Geometry: final body of the model. Coordinates: model frame, mm. Face numbers are marked on the shaded views. A direction names the side the tool comes from. Coordinates: 2 decimals unless noted, no trailing zeros. Order: outer loops, then holes, each group sorted by start corner. A loop starts at its lowest first (then second) coordinate and runs counter-clockwise, first axis right, second up. Notation, with made-up numbers: (51, 73.5) - (66, 73.5) arc R16 cw to (66, 86.5) - close; hole circle Ø11 at (-33.75, 26). An arc over 180 degrees is marked (long way). Use a Markdown table: item, result. Add a question column.
```python
from build123d import *

# Parameters (mm, degrees)
SKETCH1_W           = 50
SKETCH1_H           = 25
BOSS_EXTRUDE1_DEPTH = 25
SKETCH2_W           = 37
SKETCH2_H           = 21
CUT_EXTRUDE1_DEPTH  = 11
SKETCH3_W           = 3
SKETCH3_H           = 21
CUT_EXTRUDE2_DEPTH  = 8
SKETCH7_W           = 25
SKETCH7_H           = 25
BOSS_EXTRUDE2_DEPTH = 19
CUT_EXTRUDE3_DEPTH  = 13
SKETCH10_W          = 25
SKETCH10_H          = 25
BOSS_EXTRUDE3_DEPTH = 10
CUT_EXTRUDE5_DEPTH  = 25


with BuildPart() as part:
    # Sketch1 → Boss-Extrude1 (new body)
    with BuildSketch(Plane.XY):
        with Locations((-5, 0)):
            Rectangle(SKETCH1_W, SKETCH1_H)
    extrude(amount=BOSS_EXTRUDE1_DEPTH)

    # Sketch2 → Cut-Extrude1 (cut)
    with BuildSketch(Plane.XY.offset(25)):
        with Locations((-9.5, 0)):
            Rectangle(SKETCH2_W, SKETCH2_H)
    extrude(amount=-CUT_EXTRUDE1_DEPTH, mode=Mode.SUBTRACT)

    # Sketch3 → Cut-Extrude2 (cut)
    with BuildSketch(Plane.XY.offset(14)):
        with Locations((-1.5, 0)):
            Rectangle(SKETCH3_W, SKETCH3_H)
    extrude(amount=-CUT_EXTRUDE2_DEPTH, mode=Mode.SUBTRACT)

    # Sketch7 → Boss-Extrude2 (add)
    with BuildSketch(Plane(origin=(20, 0, 0), x_dir=(0, 0, -1), z_dir=(1, 0, 0))):
        with Locations((-12.5, 0)):
            Rectangle(SKETCH7_W, SKETCH7_H)
    extrude(amount=BOSS_EXTRUDE2_DEPTH)

    # Sketch8 → Cut-Extrude3 (cut)
    with BuildSketch(Plane.ZY.offset(-9)):
        with BuildLine():
            Line((25, -10.5), (25, 10.5))
            ThreePointArc((25, 10.5), (14.5, 0), (25, -10.5))
        make_face()
    extrude(amount=-CUT_EXTRUDE3_DEPTH, mode=Mode.SUBTRACT)

    # Sketch10 → Boss-Extrude3 (add)
    with BuildSketch(Plane(origin=(39, 0, 0), x_dir=(0, 0, -1), z_dir=(1, 0, 0))):
        with Locations((-12.5, 0)):
            Rectangle(SKETCH10_W, SKETCH10_H)
    extrude(amount=BOSS_EXTRUDE3_DEPTH)

    # Sketch9 → Cut-Extrude5 (cut)
    with BuildSketch(Plane.ZY.offset(-22)):
        with BuildLine():
            Line((25, 4), (25, -4))
            ThreePointArc((25, -4), (21, 0), (25, 4))
        make_face()
    extrude(amount=-CUT_EXTRUDE5_DEPTH, mode=Mode.SUBTRACT)


solid = part.part
```
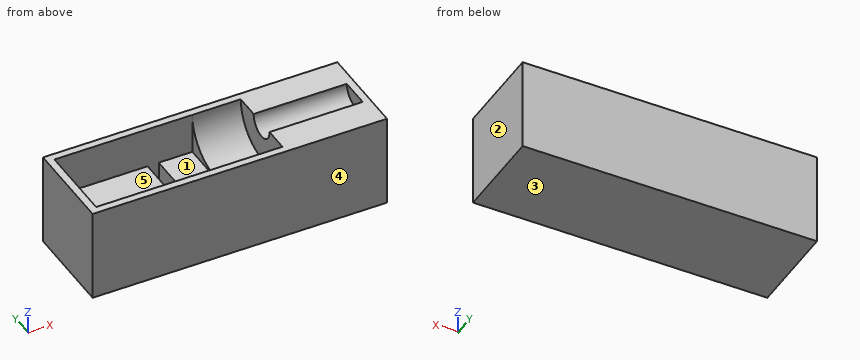
1) Ray query, line 1 along X through (y, z) = (0.25, 17.25); line 2 along X through (y, z) = (-4, 8.75); line 3 along Y through (x, z) = (1.5, 14.25). Return the intervals inside material, ascending.
2) Section B-B (y = 0). Return loops of the section in (x, z).
3) Set-up query: the marked faces 4 and 5. Return all of +Z, -Z, +X, -X, +Y, -Y with unobstructed straight access to the full face (end or side cutting, diameter ignored); none if empty.
4) Section D-D (x = 35.5). Return loops of the section in (y, z), then the cut area to 3 significant figures.
5) Section A-A (z = 8.75). Return loops of the section in (x, y).
6) Section C-C (x = 2.5). Return loops of the section in (y, z), then the cut area to 3 significant figures.
7) Pin query (flat end, axial travel): pin 1 (7 mm diameter, centred on x = 5, y = 3, fed in from +Z); pin 2 (0.9 mm diameter, centred on x = -1.5, y = -1, fed in from +Z). Return the tip coordinate at first contact, or that it passes through.
8) Draft query along X for the marked faces 1, 2 and 3. Return one class per face: pulls with the +X half, pulls with the -X half, needs draft (parallel to the pull), parting line crosses it, or undercut.
Values follow:
| question | item | result |
|---|---|---|
| 1 | line 1 | x = -30 to -28, 22 to 49 |
| 1 | line 2 | x = -30 to -3, 0 to 49 |
| 1 | line 3 | y = -12.5 to -10.5, 10.5 to 12.5 |
| 2 | outline | (-30, 0) - (49, 0) - (49, 25) - (47, 25) - (47, 21) - (22, 21) - (22, 14.5) - (9, 14.5) - (9, 14) - (0, 14) - (0, 6) - (-3, 6) - (-3, 14) - (-28, 14) - (-28, 25) - (-30, 25) - close |
| 3 | face 4 | +Z, -Z, +X, -X, -Y |
| 3 | face 5 | +Z |
| 4 | outline | (-12.5, 0) - (12.5, 0) - (12.5, 25) - (4, 25) arc R4 cw to (-4, 25) - (-12.5, 25) - close |
| 4 | area | 600 mm² |
| 5 | outline | (-30, -12.5) - (49, -12.5) - (49, 12.5) - (-30, 12.5) - close; hole (-3, -10.5) - (0, -10.5) - (0, 10.5) - (-3, 10.5) - close |
| 6 | outline | (-12.5, 0) - (12.5, 0) - (12.5, 25) - (10.5, 25) - (10.5, 14) - (-10.5, 14) - (-10.5, 25) - (-12.5, 25) - close |
| 6 | area | 394 mm² |
| 7 | pin 1 | stops at z = 14 |
| 7 | pin 2 | stops at z = 6 |
| 8 | face 1 | undercut |
| 8 | face 2 | pulls with the +X half |
| 8 | face 3 | needs draft |
